from build123d import *

# Parameters (mm, degrees)
F0_R     = 11
F0_R_2   = 5.5
F0_R_3   = 4.1
F1_DEPTH = 3
F2_DEPTH = 4.25
F3_SIZE  = 0.7
F4_R     = 0.9
F5_DEPTH = 0.5


with BuildPart() as f1:
    # F0 (on Top) → F1 (new body)
    with BuildSketch(Plane.XY):
        Circle(F0_R)
        Circle(F0_R_2, mode=Mode.SUBTRACT)
        Circle(F0_R_2)
        Circle(F0_R_3, mode=Mode.SUBTRACT)
        Circle(F0_R_3)
    extrude(amount=F1_DEPTH)

    # F0 (on Top) → F2 (join)
    with BuildSketch(Plane.XY):
        Circle(F0_R_3)
    extrude(amount=-F2_DEPTH)

    # F3
    f3_edges = [f1.edges().sort_by_distance(p)[0] for p in [
        (-4.1, 0, -4.25),
    ]]
    chamfer(f3_edges, length=F3_SIZE)

    # F4
    f4_edges = [f1.edges().sort_by_distance(p)[0] for p in [
        (11, 0, 1.5),
        (-11, 0, 0),
        (-11, 0, 3),
    ]]
    fillet(f4_edges, radius=F4_R)

    # F0 (on Top) → F5 (join)
    with BuildSketch(Plane.XY):
        Circle(F0_R_2)
        Circle(F0_R_3, mode=Mode.SUBTRACT)
    extrude(amount=-F5_DEPTH)


solid = f1.part
Geometry check sheet. Reference: the model listing, model coordinates, mm. A direction names the side the tool comes from. Give positions to 0.01 mm unless a question says otherwise; leave off trailing zeros. Order: outer loops, then holes, each group sorted by start corner. A loop starts at its lowest first (then second) coordinate and runs counter-clockwise, first axis right, second up.
1. Sectioned sample at D-D (z = 1.5). Record the boundary of the cut face in (x, y).
Completed:
outline: circle Ø22 at (0, 0)
2. Scan lines: line 1 (Z direction, x = 0.75, y = 7); line 2 (Y direction, x = 0, z = -0.75); line 3 (Z direction, x = 2.5, y = -4). Record each from-to range of solid material in increasing order.
Completed:
line 1: z = 0 to 3
line 2: y = -4.1 to 4.1
line 3: z = -0.5 to 3
3. Depth check by flat-ended pin: pin 1 (4 mm diameter, centred on y = -7, z = 0, fed in from -X). Enter the tip coordinate at first touch or a pass-through.
Completed:
pin 1: stops at x = -9.71
4. Access from +Z, -Z, +X, -X, +Y, -Y to the whole of each face (thin tool, end or side, straight path). Record for faces 1 (the face through (-0.534, 4.065, -2.004)), 2 (the face through (0, 0, -4.25)).
Completed:
face 1: -Z
face 2: -Z, +X, -X, +Y, -Y
5. Sectioned sample at C-C (z = -2). Record the boundary of the cut face in (x, y).
Completed:
outline: circle Ø8.2 at (0, 0)
6. Sectioned sample at A-A (y = 0). Record the boundary of the cut face in (x, z), then the cut area to 3 significant figures.
Completed:
outline: (-11, 0.9) arc R0.9 ccw to (-10.1, 0) - (-5.5, 0) - (-5.5, -0.5) - (-4.1, -0.5) - (-4.1, -3.55) - (-3.4, -4.25) - (3.4, -4.25) - (4.1, -3.55) - (4.1, -0.5) - (5.5, -0.5) - (5.5, 0) - (10.1, 0) arc R0.9 ccw to (11, 0.9) - (11, 2.1) arc R0.9 ccw to (10.1, 3) - (-10.1, 3) arc R0.9 ccw to (-11, 2.1) - close
area: 101 mm2
